Here's how the part is built. I have some questions about the finished solid (model axes, mm). A direction names the side the tool comes from. Give positions to 0.01 mm unless a question says otherwise; leave off trailing zeros. Write each loop counter-clockwise with the first axis right and the second up, starting at its lowest first coordinate (ties: lowest second). Pieces come first, ordered by that corner, then holes. Notation, with made-up numbers: M 1,88 L 39,88 A11 ccw 39,93 Z; hole C -10,-25 d5. An arc over 180 degrees is marked long. Use one line per item in the form item = value. Start each with the question number.
from build123d import *

# Parameters (mm, degrees)
F0_W     = 6
F0_H     = 0.3
F1_DEPTH = 7
F3_DEPTH = 2
F4_R     = 2
F5_W     = 2.3
F5_H     = 4.3
F6_DEPTH = 3.5


# Not quite as in the source:
# - a feature names something its author has since deleted; it is built from what else it names


with BuildPart() as f1:
    # F0 (on Top) → F1 (new body)
    with BuildSketch(Plane.XY):
        Polygon((0, -7), (-3.5, -0.875), (-3.5, -65.875), (-23.5, -65.875), (-23.5, -70.875), (-17.5, -70.875), (-3.6, -70.875), (-3.6, -67.775), (3.6, -67.775), (3.6, -70.875), (17.5, -70.875), (23.5, -70.875), (23.5, -65.875), (3.5, -65.875), (3.5, -0.875), align=None)
        with Locations((-20.5, -71.025)):
            Rectangle(F0_W, F0_H)
        with Locations((20.5, -71.025)):
            Rectangle(F0_W, F0_H)
        Polygon((-20, 28), (-3.5, -0.875), (0, -7), (3.5, -0.875), (20, 28), align=None)
    extrude(amount=F1_DEPTH)

    # F2 (on face) → F3 (cut)
    with BuildSketch(Plane.XY.offset(7)):
        Polygon((16.5536406433, 26), (-16.5536406433, 26), (0, -2.9688711259), align=None)
    extrude(amount=-F3_DEPTH, mode=Mode.SUBTRACT)

    # F4
    f4_edges = [f1.edges().sort_by_distance(p)[0] for p in [
        (3.5, -65.875, 3.5),
        (-3.5, -65.875, 3.5),
        (-23.5, -65.875, 3.5),
        (23.5, -65.875, 3.5),
        (-23.5, -71.175, 3.5),
        (23.5, -71.175, 3.5),
        (-20, 28, 3.5),
        (20, 28, 3.5),
        (-3.5, -0.875, 3.5),
        (3.5, -0.875, 3.5),
    ]]
    fillet(f4_edges, radius=F4_R)

    # F5 (on face) → F6 (cut)
    with BuildSketch(Plane.XY.offset(7)):
        with BuildLine():
            ThreePointArc((-1.15, -8.6188711259), (0, -9.7688711259), (1.15, -8.6188711259))
            Line((1.15, -8.6188711259), (-1.15, -8.6188711259))
        make_face()
        with Locations((0, -6.4688711259)):
            Rectangle(F5_W, F5_H)
        with BuildLine():
            Line((-1.15, -4.3188711259), (1.15, -4.3188711259))
            ThreePointArc((1.15, -4.3188711259), (0, -3.1688711259), (-1.15, -4.3188711259))
        make_face()
    extrude(amount=-F6_DEPTH, mode=Mode.SUBTRACT)


solid = f1.part
1) Suppose I cut it at D-D, the plane y = -12.5. List the corners of the cut face in (x, z) for me, and give its area (3 significant figures).
2) Will these pins go through, and if not, where does the flat tip stop? P1, Ø1.5, axis at y = -69.5, z = 3.5, coming from the +X side; P2, Ø2, axis at y = -5.5, z = 6.5, coming from the -X side; P3, Ø1, axis at x = 7, z = 6, coming from the -Y side (3 decimals); P4, Ø1, axis at y = -5.5, z = 4.5, coming from the +X side.
3) Suppose I cut it at A-A, the plane x = -10.5. List the corners of the cut face in (y, z) for me (3 decimals), and give its area (3 significant figures).
4) On a 3-axis mill with a long thin cutter (end or side, diameter ignored), from which of +Z, -Z, +X, -X, +Y, -Y can I reach the whole of each face in a straight line? I mean faces 1 (the face through (-3.6, -69, 3)), 2 (the face through (4.101, -65.305, 3.549)), 3 (the face through (1.15, -6, 5)), 4 (the face through (-3.5, -32, 3)). Say none if no direction works.
5) Please list where these lines run through material, in increasing order: line 1 (Y direction, x = 6.5, z = 6.5) (3 decimals); line 2 (Y direction, x = -14, z = 3.25) (3 decimals); line 3 (Y direction, x = 10.5, z = 6) (3 decimals).
6) Suppose I cut it at C-C, the plane z = 1.75. List the corners of the cut face in (x, y) for me (3 decimals).
7) Suppose I cut it at B-B, the plane z = 6. State how many separate pieces and enclosed holes the cut face has, and give its area (3 significant figures).
8) Thinking about a two-plate mould opening in X: for faces 5 (the face through (-20, -71.175, 3)), 6 (the face through (22.899, -70.605, 3.549)), 7 (the face through (-11.129, 12.475, 3.451)), 8 (the face through (3.6, -69, 3)), which applies, released by +X, released by -X, zero draft, split by the parting line, or undercut?
Checks:
q1.outline = M -3.5,0 L 3.5,0 L 3.5,7 L -3.5,7 Z
q1.area = 49.0 mm^2
q2.P1 = 23.5
q2.P2 = -3.5
q2.P3 = -70.875
q2.P4 = 3.5
q3.outline = M -70.875,0 L -65.875,0 L -65.875,7 L -70.875,7 Z; M 11.375,0 L 28,0 L 28,7 L 26,7 L 26,5 L 15.406,5 L 15.406,7 L 11.375,7 Z
q3.area = 130 mm^2
q4.face_1 = +Z, -Z, -Y
q4.face_2 = +Z, -Z, +X
q4.face_3 = +Z
q4.face_4 = +Z, -Z, -X
q5.line_1 = -70.875 to -65.875, 4.375 to 8.406, 26 to 28
q5.line_2 = -70.875 to -65.875, 17.5 to 28
q5.line_3 = -70.875 to -65.875, 11.375 to 15.406, 26 to 28
q6.outline = M -23.5,-69.175 A2 ccw -21.5,-71.175 L -17.5,-71.175 L -17.5,-70.875 L -3.6,-70.875 L -3.6,-67.775 L 3.6,-67.775 L 3.6,-70.875 L 17.5,-70.875 L 17.5,-71.175 L 21.5,-71.175 A2 ccw 23.5,-69.175 L 23.5,-67.875 A2 ccw 21.5,-65.875 L 5.5,-65.875 A2 cw 3.5,-63.875 L 3.5,-1.406 A2 cw 3.764,-0.414 L 18.29,25.008 A2 ccw 16.554,28 L -16.554,28 A2 ccw -18.29,25.008 L -3.764,-0.414 A2 cw -3.5,-1.406 L -3.5,-63.875 A2 cw -5.5,-65.875 L -21.5,-65.875 A2 ccw -23.5,-67.875 Z
q7.separate_pieces = 1
q7.enclosed_holes = 2
q7.area = 849 mm^2
q8.face_5 = zero draft
q8.face_6 = released by +X
q8.face_7 = released by -X
q8.face_8 = undercut
